from build123d import *

# Parameters (mm, degrees)
F1_W     = 7.6
F1_H     = 2
F3_R     = 12.9
F3_R_2   = 5.25
F4_DEPTH = 6
F5_SIZE  = 1


with BuildPart() as f2:
    # F1 (on Top) → F2 (revolve)
    with BuildSketch(Plane.XY):
        with Locations((10.2, 19.389948)):
            Rectangle(F1_W, F1_H)
        Polygon((5.25, 18.389948), (5.25, 10.389948), (14, 10.389948), (14, 18.389948), (6.4, 18.389948), align=None)
    revolve(axis=Axis((0, 1.251986, 0), (0, -1, 0)))

    # F3 (on face) → F4 (cut)
    with BuildSketch(Plane.XZ.offset(-10.389948)):
        Circle(F3_R)
        Circle(F3_R_2, mode=Mode.SUBTRACT)
    extrude(amount=-F4_DEPTH, mode=Mode.SUBTRACT)

    # F5
    f5_edges = [f2.edges().sort_by_distance(p)[0] for p in [
        (-5.25, 18.389948, 0),
    ]]
    chamfer(f5_edges, length=F5_SIZE)


solid = f2.part
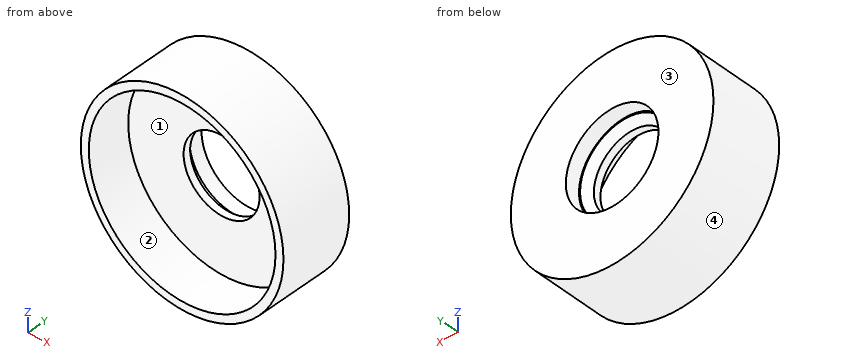
Input: part model. Units: mm. Frame: model coordinates. Face numbers are marked on the shaded views. Give positions to 0.01 mm unless a question says otherwise; leave off trailing zeros. Order: outer loops, then holes, each group sorted by start corner. A loop starts at its lowest first (then second) coordinate and runs counter-clockwise, first axis right, second up. Notation, with made-up numbers: M -29.75,85 L 24.25,85 A27 ccw 24.25,123 Z; hole C 58.5,18.25 d1. An arc over 180 degrees is marked long. Answer as a JSON object with one key per item and string values.
1. First-contact query: P1, Ø7.5, axis at x = 1, z = 3, coming from the -Y side; P2, Ø15.5, axis at x = 0, z = 0, coming from the +Y side; P3, Ø2, axis at y = 18, z = 6, coming from the +X side; P4, Ø4, axis at x = 2, z = 0, coming from the +Y side. Flat tips, straight axial feed; report the tip coordinate or a pass-through.
Result sheet:
{"P1": "y = 16.39", "P2": "y = 20.39", "P3": "x = 13.08", "P4": "through"}
2. Cut plane B-B, the plane z = 0. Output: boundary loops of the cut face in (x, y).
Result sheet:
{"outline": "M -14,10.39 L -12.9,10.39 L -12.9,16.39 L -5.25,16.39 L -5.25,17.39 L -6.25,18.39 L -6.4,18.39 L -6.4,20.39 L -14,20.39 Z; M 5.25,16.39 L 12.9,16.39 L 12.9,10.39 L 14,10.39 L 14,20.39 L 6.4,20.39 L 6.4,18.39 L 6.25,18.39 L 5.25,17.39 Z"}
3. Cut plane D-D, the plane x = -11.5. Output: boundary loops of the cut face in (y, z).
Result sheet:
{"outline": "M 10.39,-7.98 L 20.39,-7.98 L 20.39,7.98 L 10.39,7.98 L 10.39,5.84 L 16.39,5.84 L 16.39,-5.84 L 10.39,-5.84 Z"}
4. Cut plane A-A, the plane x = 0. Output: boundary loops of the cut face in (y, z).
Result sheet:
{"outline": "M 10.39,-14 L 20.39,-14 L 20.39,-6.4 L 18.39,-6.4 L 18.39,-6.25 L 17.39,-5.25 L 16.39,-5.25 L 16.39,-12.9 L 10.39,-12.9 Z; M 10.39,12.9 L 16.39,12.9 L 16.39,5.25 L 17.39,5.25 L 18.39,6.25 L 18.39,6.4 L 20.39,6.4 L 20.39,14 L 10.39,14 Z"}
5. Cut plane C-C, the plane y = 16. Output: boundary loops of the cut face in (x, z), and give its area (3 significant figures).
Result sheet:
{"outline": "C 0,0 d28; hole C 0,0 d25.8", "area": "93.0 mm²"}
6. Ray query, line 1 (Z direction, x = 0, y = 13.4); line 2 (Z direction, x = 0, y = 19); line 3 (Y direction, x = 5.25, z = -4). Return the intervals inside material, ascending. Write a range as [from, to].
Result sheet:
{"line 1": "[-14, -12.9], [12.9, 14]", "line 2": "[-14, -6.4], [6.4, 14]", "line 3": "[16.39, 20.39]"}
7. Pull-direction query (X, two-part tool) for the marked faces 1, 2, 3 and 4; classes: +X half, -X half, draft (parallel to the pull), parting line (faces both ways), or undercut.
Result sheet:
{"face 1": "undercut", "face 2": "undercut", "face 3": "draft", "face 4": "parting line"}
